```python
from build123d import *

# Parameters (mm, degrees)
BOSS_EXTRUDE1_DEPTH = 3
SKETCH2_R           = 1.5875
CUT_EXTRUDE1_DEPTH  = 3
SKETCH3_R           = 1.5875
CUT_EXTRUDE2_DEPTH  = 3


with BuildPart() as part:
    # Sketch1 → Boss-Extrude1 (new body)
    with BuildSketch(Plane(origin=(-113.226454214, -170.109741769, -309.439751514), x_dir=(0.890793361, 0, -0.454408614), z_dir=(0, -1, 0))):
        Polygon((16.200077076, -64.648683729), (51.592412285, -33.201987218), (54.382400165, 14.060345359), (22.935703655, 49.452680569), (-24.326628923, 52.242668449), (-59.718964132, 20.795971938), (-62.508952012, -26.466360639), (-31.062255502, -61.858695849), align=None)
    extrude(amount=BOSS_EXTRUDE1_DEPTH)

    # Sketch2 → Cut-Extrude1 (cut)
    with BuildSketch(Plane.XZ.offset(173.109741769)):
        with Locations((-145.375224309, -356.932300191)):
            Circle(SKETCH2_R)
        with Locations((-120.656222706, -365.870996639)):
            Circle(SKETCH2_R)
        with Locations((-165.234257313, -339.711726955)):
            Circle(SKETCH2_R)
        with Locations((-147.129073232, -267.776351499)):
            Circle(SKETCH2_R)
        with Locations((-119.068249233, -260.469800508)):
            Circle(SKETCH2_R)
        with Locations((-103.064133068, -263.787192741)):
            Circle(SKETCH2_R)
        with Locations((-84.693579832, -274.567395605)):
            Circle(SKETCH2_R)
        with Locations((-73.99225652, -286.921281828)):
            Circle(SKETCH2_R)
        with Locations((-66.685705529, -314.982105827)):
            Circle(SKETCH2_R)
    extrude(amount=-CUT_EXTRUDE1_DEPTH, mode=Mode.SUBTRACT)

    # Sketch3 → Cut-Extrude2 (cut)
    with BuildSketch(Plane(origin=(0, -170.109741769, 0), x_dir=(1, 0, 0), z_dir=(0, 1, 0))):
        with Locations((-163.939086588, 326.354614997)):
            Circle(SKETCH3_R)
        with Locations((-109.626964848, 358.226038945)):
            Circle(SKETCH3_R)
        with Locations((-75.39030048, 299.883308915)):
            Circle(SKETCH3_R)
        with Locations((-129.702422221, 268.011884967)):
            Circle(SKETCH3_R)
    extrude(amount=-CUT_EXTRUDE2_DEPTH, mode=Mode.SUBTRACT)


solid = part.part
```
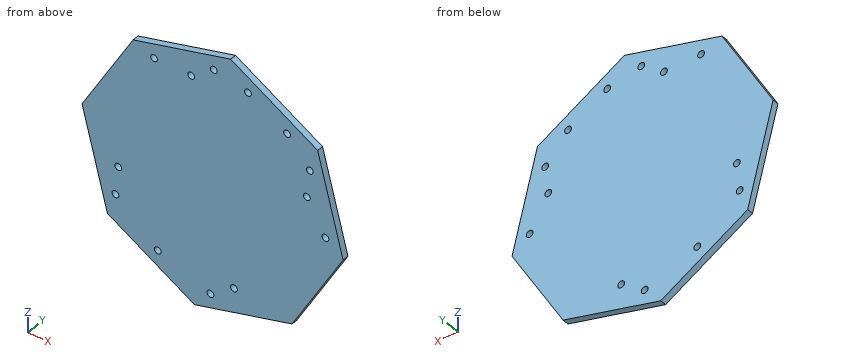
Here's how the part is built. I have some questions about the finished solid (model axes, mm). Coordinates: 2 decimals unless noted, no trailing zeros. Loops run counter-clockwise (first coordinate to the right, second up) from the corner with the lowest first, then second, coordinate; pieces in that order, holes last. Notation, with made-up numbers: (37.25, -12) -> (96.25, -12) arc R7 ccw to (96.25, 1) -> close; hole circle Ø5 at (5, 69.25). An arc over 180 degrees is marked (long way). Return JSON: item names as keys, results as strings.
1) If we section it at C-C, the plane z = -290: Write out the boundary of the cut face in (x, y).
Results below:
{"outline": "(-172.36, -173.11) -> (-66.63, -173.11) -> (-66.63, -170.11) -> (-172.36, -170.11) -> close"}
2) If we section it at A-A, the plane y = -171.05: Count the separate pieces of the cut face and the enclosed holes in it, then the cut area to 3 significant figures.
Results below:
{"separate pieces": "1", "enclosed holes": "13", "area": "10,700 mm²"}
3) I need wall thicknesses on line 1 (Z direction, x = -146, y = -170.25); line 2 (Z direction, x = -130, y = -172.15); line 3 (X direction, y = -170.45, z = -316). Which ranges of each line are inside material? Lowest first, please. Write a range as from..to.
Results below:
{"line 1": "-363.93..-358.39, -355.47..-268.89, -266.66..-260.92", "line 2": "-373.32..-269.57, -266.45..-256.75", "line 3": "-177.97..-67.9, -65.47..-59.86"}
4) Will these pins go through, and if not, where does the flat tip stop? pin 1 (1.5 mm diameter, centred on x = -88, y = -172.5, fed in from +Z); pin 2 (2.5 mm diameter, centred on x = -119.07, z = -260.47, fed in from +Y); pin 3 (1.5 mm diameter, centred on y = -172, z = -291.5, fed in from +X).
Results below:
{"pin 1": "z = -265", "pin 2": "through", "pin 3": "x = -66.04"}
5) If we section it at B-B, the plane x = -125: Write out the boundary of the cut face in (y, z), then the cut area to 3 significant figures.
Results below:
{"outline": "(-173.11, -373.56) -> (-170.11, -373.56) -> (-170.11, -255.45) -> (-173.11, -255.45) -> close", "area": "354 mm²"}
